Can you work these out from the model? Positions are in its coordinate system, mm. Face numbers are marked on the shaded views. A direction names the side the tool comes from. Round coordinates to 2 decimals unless told otherwise and drop trailing zeros. Loops run counter-clockwise (first coordinate to the right, second up) from the corner with the lowest first, then second, coordinate; pieces in that order, holes last. Notation, with made-up numbers: M 5.25,78 L 46.25,78 A20 cw 46.25,92 Z; hole C -35.75,-6.75 d1. An arc over 180 degrees is marked long. Return JSON: item names as keys, results as strings.
```python
from build123d import *

# Parameters (mm, degrees)
SKETCH1_W           = 39
SKETCH1_H           = 26
BOSS_EXTRUDE1_DEPTH = 15
SKETCH2_W           = 39
SKETCH2_H           = 26
SKETCH2_W_2         = 35
SKETCH2_H_2         = 22
CUT_EXTRUDE1_DEPTH  = 8.5
FILLET1_R           = 5
SKETCH3_R           = 19.5
BOSS_EXTRUDE2_DEPTH = 120
BOSS_EXTRUDE3_DEPTH = 15
FILLET2_R           = 25
FILLET3_R           = 35


with BuildPart() as part:
    # Sketch1 → Boss-Extrude1 (new body)
    with BuildSketch(Plane.XY):
        Rectangle(SKETCH1_W, SKETCH1_H)
    extrude(amount=BOSS_EXTRUDE1_DEPTH)

    # Sketch2 → Cut-Extrude1 (cut)
    with BuildSketch(Plane.XY.offset(15)):
        Rectangle(SKETCH2_W, SKETCH2_H)
        Rectangle(SKETCH2_W_2, SKETCH2_H_2, mode=Mode.SUBTRACT)
    extrude(amount=-CUT_EXTRUDE1_DEPTH, mode=Mode.SUBTRACT)

    # Fillet1
    fillet1_edges = [part.edges().sort_by_distance(p)[0] for p in [
        (19.5, -13, 3.25),
        (-19.5, -13, 3.25),
        (-19.5, 13, 3.25),
        (19.5, 13, 3.25),
        (17.5, -11, 10.75),
        (17.5, 11, 10.75),
        (-17.5, 11, 10.75),
        (-17.5, -11, 10.75),
    ]]
    fillet(fillet1_edges, radius=FILLET1_R)

    # Sketch3 → Boss-Extrude2 (add)
    with BuildSketch(Plane.XY.offset(15)):
        Circle(SKETCH3_R)
    extrude(amount=BOSS_EXTRUDE2_DEPTH)

    # Sketch4 → Boss-Extrude3 (add, symmetric)
    with BuildSketch(Plane(origin=(0, 0, 0), x_dir=(0, 0, -1), z_dir=(1, 0, 0))):
        Polygon((-135, 19.5), (-135, -19.5), (-135, -60), (-935, -60), (-935, 60), (-135, 60), align=None)
    extrude(amount=BOSS_EXTRUDE3_DEPTH, both=True)

    # Fillet2
    fillet2_edges = [part.edges().sort_by_distance(p)[0] for p in [
        (0, 60, 935),
    ]]
    fillet(fillet2_edges, radius=FILLET2_R)

    # Fillet3
    fillet3_edges = [part.edges().sort_by_distance(p)[0] for p in [
        (0, -60, 935),
    ]]
    fillet(fillet3_edges, radius=FILLET3_R)


solid = part.part
```
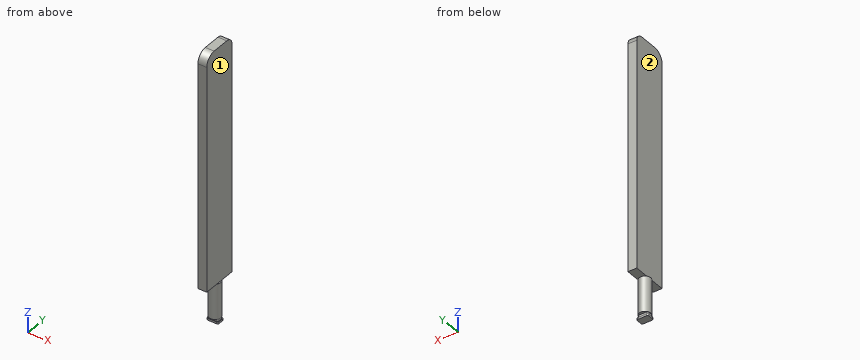
Q1. If I drill on line 1 along X through (y, z) = (-49, 884); line 2 along Z through (x, y) = (-3.5, 17.5); line 3 along Z through (x, y) = (6, 29.5), over which ranges is the centre line in solid material (lowest first)?
Results:
{"line 1": "x = -15 to 15", "line 2": "z = 15 to 935", "line 3": "z = 135 to 935"}
Q2. On a 3-axis mill with a long thin cutter (end or side, diameter ignored), from which of +Z, -Z, +X, -X, +Y, -Y can I reach the whole of each face in a straight line? I mean the marked faces 1 and 2. Say none if no direction works.
Results:
{"face 1": "+Z, +X, +Y, -Y", "face 2": "+Z, -X, +Y, -Y"}
Q3. Suppose I cut it at B-B, the plane z = 645. Please give me the cut outline in (x, y), plus the area to 3 significant figures.
Results:
{"outline": "M -15,-60 L 15,-60 L 15,60 L -15,60 Z", "area": "3,600 mm2"}
Q4. Suppose I cut it at D-D, the plane z = 67. Please give me the cut outline in (x, y), plus the area to 3 significant figures.
Results:
{"outline": "C 0,0 d39", "area": "1,190 mm2"}
Q5. I'm going to push flat-ended pins straight in: pin 1 Ø2.5 at (y, z) = (2.5, 12.5) entering from -X; pin 2 Ø9 at (x, y) = (-1, 41) entering from -Z; pin 3 Ø1.3 at (x, y) = (-18, -4) entering from +Z. Where does each tip first touch, or does it pass through?
Results:
{"pin 1": "stops at x = -17.5", "pin 2": "stops at z = 135", "pin 3": "stops at z = 135"}
Q6. Suppose I cut it at C-C, the plane y = -49.5. Please give me the cut outline in (x, z) (3 decimals).
Results:
{"outline": "M -15,135 L 15,135 L 15,924.995 L -15,924.995 Z"}
Q7. Suppose I cut it at A-A, the plane x = 0. Please give me the cut outline in (y, z), plus the area to 3 significant figures.
Results:
{"outline": "M -60,135 L -19.5,135 L -19.5,15 L -11,15 L -11,6.5 L -13,6.5 L -13,0 L 13,0 L 13,6.5 L 11,6.5 L 11,15 L 19.5,15 L 19.5,135 L 60,135 L 60,910 A25 ccw 35,935 L -25,935 A35 ccw -60,900 Z", "area": "101,000 mm2"}
